```python
from build123d import *

# Parameters (mm, degrees)
IZIM1_R                     = 25
IZIM1_R_2                   = 16
Y_KSEKLIK_EKSTR_ZYON1_DEPTH = 45
Y_KSEKLIK_EKSTR_ZYON2_DEPTH = 35
Y_KSEKLIK_EKSTR_ZYON4_START = -10
Y_KSEKLIK_EKSTR_ZYON4_DEPTH = 10
RADYUS2_R                   = 6
IZIM6_R                     = 10
Y_KSEKLIK_EKSTR_ZYON6_DEPTH = 10
IZIM7_R                     = 19
IZIM7_R_2                   = 10
Y_KSEKLIK_EKSTR_ZYON7_DEPTH = 8
RADYUS3_R                   = 25
AYNALAMA1_START             = -45
AYNALAMA1_OUTLINE_R         = 10
AYNALAMA1_DEPTH             = 10
AYNALAMA1_START_2           = -48
AYNALAMA1_2_OUTLINE_R       = 19
AYNALAMA1_2_OUTLINE_R_2     = 10
AYNALAMA1_2_DEPTH           = 16
IZIM8_R                     = 5
KES_EKSTR_ZYON1_DEPTH       = 16


# Read off the part's stored shape, not the designer's step: Aynalama1
# Some blends are built 0.0001 mm under size
with BuildPart() as part:
    # Çizim1 → Yükseklik-Ekstrüzyon1 (new body)
    with BuildSketch(Plane.XY):
        Circle(IZIM1_R)
        Circle(IZIM1_R_2, mode=Mode.SUBTRACT)
    extrude(amount=-Y_KSEKLIK_EKSTR_ZYON1_DEPTH)

    # Çizim4 → Yükseklik-Ekstrüzyon2 (add)
    with BuildSketch(Plane.XY.offset(-10)):
        with BuildLine():
            Line((25, 0), (25, 22))
            ThreePointArc((25, 22), (25.878679656, 24.121320344), (28, 25))
            Line((28, 25), (33, 25))
            ThreePointArc((33, 25), (41.485281374, 28.514718626), (45, 37))
            Line((45, 37), (45, 44))
            ThreePointArc((45, 44), (46.757359313, 48.242640687), (51, 50))
            Line((51, 50), (75, 50))
            Line((75, 50), (75, 60))
            Line((75, 60), (35, 60))
            Line((35, 60), (35, 38))
            ThreePointArc((35, 38), (34.121320344, 35.878679656), (32, 35))
            Line((32, 35), (-32, 35))
            ThreePointArc((-32, 35), (-34.121320344, 35.878679656), (-35, 38))
            Line((-35, 38), (-35, 60))
            Line((-35, 60), (-75, 60))
            Line((-75, 60), (-75, 50))
            Line((-75, 50), (-51, 50))
            ThreePointArc((-51, 50), (-46.757359313, 48.242640687), (-45, 44))
            Line((-45, 44), (-45, 37))
            ThreePointArc((-45, 37), (-41.485281374, 28.514718626), (-33, 25))
            Line((-33, 25), (-28, 25))
            ThreePointArc((-28, 25), (-25.878679656, 24.121320344), (-25, 22))
            Line((-25, 22), (-25, 0))
            ThreePointArc((-25, 0), (0, 25), (25, 0))
        make_face()
    extrude(amount=-Y_KSEKLIK_EKSTR_ZYON2_DEPTH)

    # Çizim5 → Yükseklik-Ekstrüzyon4 (add)
    with BuildSketch(Plane(origin=(0, 0, -45), x_dir=(-1, 0, 0), z_dir=(0, 0, -1)).offset(Y_KSEKLIK_EKSTR_ZYON4_START)):
        with BuildLine():
            Line((69, 50), (69, 18))
            ThreePointArc((69, 18), (67.242640687, 13.757359313), (63, 12))
            Line((63, 12), (57, 12))
            ThreePointArc((57, 12), (48.514718626, 8.485281374), (45, 0))
            Line((45, 0), (45, -28))
            Line((45, -28), (-45, -28))
            Line((-45, -28), (-45, 0))
            ThreePointArc((-45, 0), (-48.514718626, 8.485281374), (-57, 12))
            Line((-57, 12), (-63, 12))
            ThreePointArc((-63, 12), (-67.242640687, 13.757359313), (-69, 18))
            Line((-69, 18), (-69, 50))
            Line((-69, 50), (-51, 50))
            ThreePointArc((-51, 50), (-46.757359313, 48.242640687), (-45, 44))
            Line((-45, 44), (-45, 37))
            ThreePointArc((-45, 37), (-41.485281374, 28.514718626), (-33, 25))
            Line((-33, 25), (-28, 25))
            ThreePointArc((-28, 25), (-25.878679656, 24.121320344), (-25, 22))
            Line((-25, 22), (-25, 0))
            ThreePointArc((-25, 0), (0, -25), (25, 0))
            Line((25, 0), (25, 22))
            ThreePointArc((25, 22), (25.878679656, 24.121320344), (28, 25))
            Line((28, 25), (33, 25))
            ThreePointArc((33, 25), (41.485281374, 28.514718626), (45, 37))
            Line((45, 37), (45, 44))
            ThreePointArc((45, 44), (46.757359313, 48.242640687), (51, 50))
            Line((51, 50), (69, 50))
        make_face()
    extrude(amount=Y_KSEKLIK_EKSTR_ZYON4_DEPTH)

    # Radyus2
    radyus2_edges = [part.edges().sort_by_distance(p)[0] for p in [
        (-69, 50, -40),
        (69, 50, -40),
    ]]
    fillet(radyus2_edges, radius=RADYUS2_R - 0.0001)  # a hair under: the kernel refuses the full size

    # Çizim6 → Yükseklik-Ekstrüzyon6 (add)
    with BuildSketch(Plane(origin=(45, 0, 0), x_dir=(0, 0, -1), z_dir=(1, 0, 0))):
        with BuildLine():
            Line((45, -28), (103.939212458, -18.771282059))
            ThreePointArc((103.939212458, -18.771282059), (120, 0), (103.939212458, 18.771282059))
            Line((103.939212458, 18.771282059), (45, 28))
            Line((45, 28), (45, -28))
        make_face()
        with Locations((101, 0)):
            Circle(IZIM6_R, mode=Mode.SUBTRACT)
    extrude(amount=-Y_KSEKLIK_EKSTR_ZYON6_DEPTH)

    # Çizim7 → Yükseklik-Ekstrüzyon7 (add, symmetric)
    with BuildSketch(Plane(origin=(40, 0, 0), x_dir=(0, 0, -1), z_dir=(1, 0, 0))):
        with Locations((101, 0)):
            Circle(IZIM7_R)
        with Locations((101, 0)):
            Circle(IZIM7_R_2, mode=Mode.SUBTRACT)
    extrude(amount=Y_KSEKLIK_EKSTR_ZYON7_DEPTH, both=True)

    # Radyus3
    # the kernel refuses this fillet: 25 mm, written as the material it adds along each edge
    with BuildSketch(Plane(origin=(45, 28, -45), x_dir=(0, 1, 0), z_dir=(-1, 0, 0))) as radyus3_piece_1:
        with BuildLine():
            CenterArc((RADYUS3_R * 0.855604187922, RADYUS3_R), RADYUS3_R, 188.899130451, 81.100869549)
            Line((-RADYUS3_R * 0.132358025694, RADYUS3_R * 0.845304607478), (0, 0))
            Line((0, 0), (RADYUS3_R * 0.855604187922, 0))
        make_face()
    extrude(amount=10)

    # Aynalama1 outline → Aynalama1 (add)
    with BuildSketch(Plane.YZ.offset(AYNALAMA1_START)):
        with BuildLine():
            ThreePointArc((-18.771282059, -103.939212458), (0, -120), (18.771282059, -103.939212458))
            Line((18.771282059, -103.939212458), (24.691049358, -66.132615187))
            ThreePointArc((24.691049358, -66.132615187), (33.137176044, -51.004150186), (49.390104698, -45))
            Line((49.390104698, -45), (-28, -45))
            Line((-28, -45), (-18.771282059, -103.939212458))
        make_face()
        with Locations((0, -101)):
            Circle(AYNALAMA1_OUTLINE_R, mode=Mode.SUBTRACT)
    extrude(amount=AYNALAMA1_DEPTH)

    # Aynalama1 2 outline → Aynalama1 2 (add)
    with BuildSketch(Plane.YZ.offset(AYNALAMA1_START_2)):
        with Locations((0, -101)):
            Circle(AYNALAMA1_2_OUTLINE_R)
        with Locations((0, -101)):
            Circle(AYNALAMA1_2_OUTLINE_R_2, mode=Mode.SUBTRACT)
    extrude(amount=AYNALAMA1_2_DEPTH)

    # Çizim8 → Kes-Ekstrüzyon1 (cut)
    with BuildSketch(Plane.XZ.offset(-50)):
        with Locations((63, -22)):
            Circle(IZIM8_R)
        with Locations(Location((-63, -22, 0), (0, 0, 90))):
            Circle(IZIM8_R)
    extrude(amount=-KES_EKSTR_ZYON1_DEPTH, mode=Mode.SUBTRACT)


solid = part.part
```
Geometry: final body of the model. Coordinates: model frame, mm. A direction names the side the tool comes from. Coordinates: 2 decimals unless noted, no trailing zeros. Order: outer loops, then holes, each group sorted by start corner. A loop starts at its lowest first (then second) coordinate and runs counter-clockwise, first axis right, second up. Notation, with made-up numbers: (56, 23) -> (68, 23) arc R25 cw to (68, 44) -> close; hole circle Ø10 at (75.25, 10.25). An arc over 180 degrees is marked (long way). Use CSV: the item, a comma, the result in double quotes.
1) Section B-B on x = 0. Output: boundary loops of the cut face in (y, z), then the cut area to 3 significant figures.
Findings:
outline,"(-28, -45) -> (-16, -45) -> (-16, 0) -> (-25, 0) -> (-25, -35) -> (-28, -35) -> close; (16, -45) -> (35, -45) -> (35, -10) -> (25, -10) -> (25, 0) -> (16, 0) -> close"
area,"1,190 mm^2"
2) Mould query, pull axis X, two halves, no side actions, for faces 4 (the cylindrical face through (40.07, 32.95, -51.166)), 5 (the flat face through (-45, 2, -61)), 6 (the flat face through (32, -8, -109)). Classes: +X half, -X half, draft (parallel to the pull), parting line (faces both ways), or undercut.
Findings:
face 4,"draft"
face 5,"-X half"
face 6,"undercut"
3) Pin query (flat end, axial travel): pin 1 Ø7 at (x, z) = (63.5, -34.5) entering from -Y; pin 2 Ø7.5 at (y, z) = (40, -16.5) entering from +X; pin 3 Ø17.5 at (y, z) = (8.5, -23.5) entering from -X. Return the tip coordinate at first contact, or that it passes through.
Findings:
pin 1,"stops at y = 12"
pin 2,"stops at x = 45"
pin 3,"stops at x = -25"
4) Section C-C on z = -78. Output: boundary loops of the cut face in (x, y).
Findings:
outline,"(-45, -22.83) -> (-35, -22.83) -> (-35, 22.83) -> (-45, 22.83) -> close; (35, -22.83) -> (45, -22.83) -> (45, 22.83) -> (35, 22.83) -> close"
5) Access query for faces 1 (the flat face through (0, 35, -27)), 2 (the flat face through (25, 11, -22)), 3 (the flat face through (32, 12, -35)). Directions: +Z, -Z, +X, -X, +Y, -Y. A direction counts if a zero-diameter tool reaches every point of the face in a straight line with its end or side. Return the directions, or none.
Findings:
face 1,"+Z, -Z, +Y"
face 2,"+Z, +X, -Y"
face 3,"+Z, -Y"
6) Line query: line 1 (Y direction, x = 0, z = -24.5); line 2 (X direction, y = 6, z = -77); line 3 (X direction, y = -13, z = -101.5). Output: solid intervals per line, ascending.
Findings:
line 1,"y = -25 to -16, 16 to 35"
line 2,"x = -45 to -35, 35 to 45"
line 3,"x = -48 to -32, 32 to 48"
7) Section A-A on z = -22. State how many separate pieces and enclosed holes the cut face has, then the cut area to 3 significant figures.
Findings:
separate pieces,"3"
enclosed holes,"1"
area,"3,190 mm^2"
8) Section D-D on y = -14. Output: boundary loops of the cut face in (x, z), then the cut area to 3 significant figures.
Findings:
outline,"(-48, -113.85) -> (-32, -113.85) -> (-32, -88.15) -> (-35, -88.15) -> (-35, -45) -> (-7.75, -45) -> (-7.75, 0) -> (-20.71, 0) -> (-20.71, -35) -> (-45, -35) -> (-45, -88.15) -> (-48, -88.15) -> close; (7.75, -45) -> (35, -45) -> (35, -88.15) -> (32, -88.15) -> (32, -113.85) -> (48, -113.85) -> (48, -88.15) -> (45, -88.15) -> (45, -35) -> (20.71, -35) -> (20.71, 0) -> (7.75, 0) -> close"
area,"3,340 mm^2"
